```python
from build123d import *

# Parameters (mm, degrees)
F0_R     = 20
F0_R_2   = 10
F1_DEPTH = 28
F2_DEPTH = 12
F3_DEPTH = 40


# Not quite as in the source:
# - ends of sketch curves that miss each other by under 0.0002 mm in the source are joined


with BuildPart() as f1:
    # F0 (on Front) → F1 (new body)
    with BuildSketch(Plane.XZ):
        with Locations((0, 32)):
            Circle(F0_R)
        with Locations((0, 32)):
            Circle(F0_R_2, mode=Mode.SUBTRACT)
    extrude(amount=F1_DEPTH)

    # F0 (on Front) → F2 (join)
    with BuildSketch(Plane.XZ):
        with BuildLine():
            add(Edge.make_bspline(
                [(-43.9999970173, -38), (-43.9999970173, -14.6666666667), (-43.9999970173, 8.6666666667), (-43.9999970173, 32)],
                knots=[0, 0, 0, 0, 70, 70, 70, 70], degree=3))
            Line((-43.9999970173, -38), (44, -38))
            Line((44, -38), (44, 32))
            ThreePointArc((44, 32), (0, 76), (-43.9999970173, 32))
        make_face()
        with Locations((0, 32)):
            Circle(F0_R, mode=Mode.SUBTRACT)
    extrude(amount=F2_DEPTH)

    # F0 (on Front) → F3 (join)
    with BuildSketch(Plane.XZ):
        Polygon((-43.9999970173, -38), (-43.9999970173, -68), (-20, -68), (-20, -53), (20, -53), (20, -68), (44, -68), (44, -38), align=None)
    extrude(amount=F3_DEPTH)


solid = f1.part
```
Design review of the part built by this model. Coordinates are the model's own, in mm. A direction names the side the tool comes from. Round coordinates to 2 decimals unless told otherwise and drop trailing zeros. Order: outer loops, then holes, each group sorted by start corner. A loop starts at its lowest first (then second) coordinate and runs counter-clockwise, first axis right, second up. Notation, with made-up numbers: (46.5, 52) - (72.5, 52) arc R22 cw to (72.5, 79) - close; hole circle Ø9 at (61.5, -13.75). An arc over 180 degrees is marked (long way). One line per question, with ' | ' between items.
Item 1: Take a section at B-B, the plane x = 0. Write out the cut boundary in (y, z), then the cut area to 3 significant figures.
Checks:
outline: (-40, -53) - (0, -53) - (0, 22) - (-28, 22) - (-28, 12) - (-12, 12) - (-12, -38) - (-40, -38) - close; (-28, 42) - (0, 42) - (0, 76) - (-12, 76) - (-12, 52) - (-28, 52) - close | area: 2,050 mm²
Item 2: Take a section at C-C, the plane z = -32. Write out the cut boundary in (x, y), then the cut area to 3 significant figures.
Checks:
outline: (-44, -12) - (44, -12) - (44, 0) - (-44, 0) - close | area: 1,060 mm²
Item 3: Take a section at D-D, the plane x = 12.5. Write out the cut boundary in (y, z).
Checks:
outline: (-40, -53) - (0, -53) - (0, 74.19) - (-12, 74.19) - (-12, 47.61) - (-28, 47.61) - (-28, 16.39) - (-12, 16.39) - (-12, -38) - (-40, -38) - close
Item 4: Draft analysis for pull direction X (two halves, no side actions). For faces 1 (the face through (1, -12, 7)), 2 (the face through (44, -11, -30)), 3 (the face through (-20, -20, -61)), state which applies: +X half, -X half, draft (parallel to the pull), parting line (faces both ways), or undercut.
Checks:
face 1: draft | face 2: +X half | face 3: undercut
Item 5: Wall thickness on line 1 (Z direction, x = 0, y = -22); line 2 (X direction, y = -10.5, z = -58.5); line 3 (Z direction, x = 0, y = -10.75): over which ranges is each line inside the solid? List them lowest first. Write a range as [from, to].
Checks:
line 1: [-53, -38], [12, 22], [42, 52] | line 2: [-44, -20], [20, 44] | line 3: [-53, 22], [42, 76]
Item 6: Machinability: for faces 4 (the face through (0, -20, -53)), 5 (the face through (-5, -28, 41)), 6 (the face through (-2.6, -19.89, 51.83)), 7 (the face through (1, -26, -38)), 8 (the face through (0.97, -5.92, 75.99)), which of the approach directions +Z, -Z, +X, -X, +Y, -Y give a long, thin tool a straight path to every point of the face, cutting with its end or side? Answer none if there is none.
Checks:
face 4: -Z, +Y, -Y | face 5: +Z, +X, -X, -Y | face 6: -Y | face 7: +X, -X, -Y | face 8: +Z, +Y, -Y
Item 7: Take a section at A-A, the plane y = -13.5. Write out the cut boundary in (x, z), then the cut area to 3 significant figures.
Checks:
outline: (-44, -68) - (-20, -68) - (-20, -53) - (20, -53) - (20, -68) - (44, -68) - (44, -38) - (-44, -38) - close; circle Ø40 at (0, 32); hole circle Ø20 at (0, 32) | area: 2,980 mm²
Item 8: For P1, Ø12, axis at x = -4.5, z = 28, coming from the -Y side; P2, Ø10, axis at x = 18, y = -13, coming from the +Z side; P3, Ø12, axis at x = 6.5, y = -17.5, coming from the -Z side, all flat-tipped, find the tip position at first contact; note any pin that passes through.
Checks:
P1: y = -28 | P2: z = 74 | P3: z = -53
